```python
from build123d import *

# Parameters (mm, degrees)
SKETCH1_W           = 76
SKETCH1_H           = 70
BOSS_EXTRUDE1_DEPTH = 88.3
SKETCH2_R           = 31
BOSS_EXTRUDE2_DEPTH = 6.2
CIRPATTERN1_COUNT   = 6
SKETCH8_R           = 23.588802374
CUT_EXTRUDE1_DEPTH  = 11.11


with BuildPart() as part:
    # Sketch1 → Boss-Extrude1 (new body)
    with BuildSketch(Plane(origin=(0, 0, 0), x_dir=(1, 0, 0), z_dir=(0, 1, 0))):
        Rectangle(SKETCH1_W, SKETCH1_H)
    extrude(amount=BOSS_EXTRUDE1_DEPTH)

    # Sketch2 → Boss-Extrude2 (add)
    with BuildSketch(Plane(origin=(0, 88.3, 0), x_dir=(1, 0, 0), z_dir=(0, 1, 0))):
        Circle(SKETCH2_R)
    extrude(amount=BOSS_EXTRUDE2_DEPTH)

    # Sketch7 → M3x0.5 Tapped Hole3 (revolve, cut)
    with BuildSketch(Plane(origin=(27, 94.5, 0), x_dir=(0, 0, 1), z_dir=(1, 0, 0))):
        Polygon((0, 0), (0, 7.251075774), (1.25, 6.5), (1.25, 0), align=None)
    m3x0_5_tapped_hole3 = revolve(axis=Axis((27, 100.85, 0), (0, -1, 0)), mode=Mode.SUBTRACT)

    # CirPattern1: M3x0.5 Tapped Hole3 ×6 about axis
    cirpattern1_axis = Axis((0, 0, 0), (0, 1, 0))
    for i in range(1, CIRPATTERN1_COUNT):
        add(m3x0_5_tapped_hole3.rotate(cirpattern1_axis, i * 360 / CIRPATTERN1_COUNT), mode=Mode.SUBTRACT)

    # Sketch8 → Cut-Extrude1 (cut)
    with BuildSketch(Plane(origin=(0, 94.5, 0), x_dir=(1, 0, 0), z_dir=(0, 1, 0))):
        Circle(SKETCH8_R)
    extrude(amount=-CUT_EXTRUDE1_DEPTH, mode=Mode.SUBTRACT)


solid = part.part
```
Work out the finished part from the listing and answer in its coordinate system (mm). A direction names the side the tool comes from. Give positions to 0.01 mm unless a question says otherwise; leave off trailing zeros. Loops run counter-clockwise (first coordinate to the right, second up) from the corner with the lowest first, then second, coordinate; pieces in that order, holes last. Notation, with made-up numbers: (65.5, 36) -> (106.5, 36) arc R14 ccw to (106.5, 49) -> close; hole circle Ø4 at (78.5, 55.25). An arc over 180 degrees is marked (long way). One line per question, with ' | ' between items. Start each with the question number.
1) Section C-C, the plane z = 27.5 is taken. Determine the outline of the cut face in (x, y), then the cut area to 3 significant figures.
2) Each of these flat-tipped pins is pushed along its axis until it touches: pin 1 (3 mm diameter, centred on x = 3.5, z = 4, fed in from +Y); pin 2 (1.5 mm diameter, centred on x = -27, z = 0, fed in from +Y). Where does it stop, or does it pass through?
3) Section B-B, the plane z = 6 is taken. Determine the outline of the cut face in (x, y).
4) Straight lines are drawn through the part: L1, parallel to X at y = 89.5, z = 0; L2, parallel to Z at x = -13, y = 89; L3, parallel to Y at x = -31, z = -6. For each, find the intervals that lie inside material, in ascending order.
5) Section A-A, the plane x = 0 is taken. Determine the outline of the cut face in (y, z), then the cut area to 3 significant figures.
6) For faces 1 (the face through (-38, 44, 0)), 2 (the face through (-28.22, 91.3, 0.27)), determine the directions among +Z, -Z, +X, -X, +Y, -Y from which every point of the face is accessible in a straight line to the end or side of a thin tool.
Resolved:
1) outline: (-38, 0) -> (38, 0) -> (38, 88.3) -> (14.31, 88.3) -> (14.31, 94.5) -> (-14.31, 94.5) -> (-14.31, 88.3) -> (-38, 88.3) -> close | area: 6,890 mm2
2) pin 1: y = 83.39 | pin 2: y = 87.7
3) outline: (-38, 0) -> (38, 0) -> (38, 88.3) -> (30.41, 88.3) -> (30.41, 94.5) -> (22.81, 94.5) -> (22.81, 83.39) -> (-22.81, 83.39) -> (-22.81, 94.5) -> (-30.41, 94.5) -> (-30.41, 88.3) -> (-38, 88.3) -> close
4) L1: -31 to -28.25, -25.75 to -23.59, 23.59 to 25.75, 28.25 to 31 | L2: -28.14 to -24.53, -22.24 to -19.68, 19.68 to 22.24, 24.53 to 28.14 | L3: 0 to 88.3
5) outline: (0, -35) -> (88.3, -35) -> (88.3, -31) -> (94.5, -31) -> (94.5, -23.59) -> (83.39, -23.59) -> (83.39, 23.59) -> (94.5, 23.59) -> (94.5, 31) -> (88.3, 31) -> (88.3, 35) -> (0, 35) -> close | area: 6,040 mm2
6) face 1: +Z, -Z, -X, +Y, -Y | face 2: +Y
